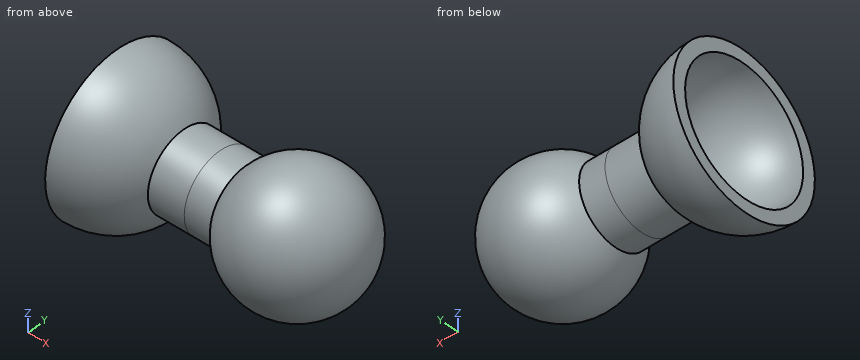
from build123d import *

# Parameters (mm, degrees)
SALIENTE_EXTRUIR2_START             = -40
CROQUIS2_R                          = 15
SALIENTE_EXTRUIR2_DEPTH             = 10
SALIENTE_EXTRUIR2_DIRECTION_2_REACH = 93.962


with BuildPart() as part:
    # Croquis1 → Revolución-Lámina1 (revolve)
    with BuildSketch(Plane(origin=(0, 0, 0), x_dir=(1, 0, 0), z_dir=(0, 1, 0))):
        with BuildLine():
            ThreePointArc((25, 0), (17.67766953, 17.67766953), (0, 25))
            Line((0, 25), (0, 30))
            ThreePointArc((0, 30), (21.213203436, 21.213203436), (30, 0))
            Line((30, 0), (25, 0))
        make_face()
    revolve(axis=Axis((0, 0, 0), (1, 0, 0)))

    # Croquis2 → Saliente-Extruir2 (add)
    with BuildSketch(Plane.ZY.offset(SALIENTE_EXTRUIR2_START)):
        Circle(CROQUIS2_R)
    extrude(amount=-SALIENTE_EXTRUIR2_DEPTH)

    # Croquis2 → Saliente-Extruir2 direction 2 (add, up to next)
    with BuildSketch(Plane.ZY.offset(SALIENTE_EXTRUIR2_START), mode=Mode.PRIVATE) as saliente_extruir2_direction_2_sk1:
        Circle(CROQUIS2_R)
    saliente_extruir2_direction_2_tool1 = extrude(saliente_extruir2_direction_2_sk1.sketch, amount=SALIENTE_EXTRUIR2_DIRECTION_2_REACH, mode=Mode.PRIVATE) - part.part
    add(saliente_extruir2_direction_2_tool1.solids().sort_by_distance((40, 0, 0))[0])

    # Croquis3 → Revolución1 (revolve)
    with BuildSketch(Plane.XY, mode=Mode.PRIVATE) as revoluci_n1_sk:
        with BuildLine():
            Line((50, 0), (50, 15))
            ThreePointArc((50, 15), (77.90569415, 23.717082451), (95, 0))
            Line((95, 0), (50, 0))
        make_face()
    revolve(revoluci_n1_sk.sketch.rotate(Axis((50, 0, 0), (1, 0, 0)), 90), axis=Axis((50, 0, 0), (1, 0, 0)))


solid = part.part
Source: CAD feature listing. Evaluate the final solid. Frame: model axes, mm. Round coordinates to 2 decimals unless told otherwise and drop trailing zeros. Loops run counter-clockwise (first coordinate to the right, second up) from the corner with the lowest first, then second, coordinate; pieces in that order, holes last. Notation, with made-up numbers: (16.5, -12.5) - (64.5, -12.5) arc R20 ccw to (64.5, -3.5) - close; hole circle Ø8 at (53.25, 13.25). An arc over 180 degrees is marked (long way). Write item = value, one per line. Start each with the question number.
(1) Section query C-C, the plane z = 20.5. Output: boundary loops of the cut face in (x, y).
(2) Section query D-D, the plane y = -17. Output: boundary loops of the cut face in (x, z), plus the area to 3 significant figures.
(3) Pin query (flat end, axial travel): pin 1 (5 mm diameter, centred on x = 28, y = 13, fed in from +Z); pin 2 (1 mm diameter, centred on y = -13.5, z = 18, fed in from -X); pin 3 (8 mm diameter, centred on x = 75, z = -12.5, fed in from -Y). Return the tip coordinate at first contact, or that it passes through.
(4) Section query A-A, the plane y = 0. Output: boundary loops of the cut face in (x, z), plus the area to 3 significant figures.
(5) Ray query, line 1 along X through (y, z) = (-17, -1); line 2 along Y through (x, z) = (8, -20.5); line 3 along X through (y, z) = (-16.5, 7.5). Return the intervals inside material, ascending. Write a range as from..to.
Conclusion:
q1.outline = (0, -21.9) arc R21.9 ccw to (0, 21.9) - (0, 14.31) arc R14.31 cw to (0, -14.31) - close; circle Ø28.62 at (70, 0)
q2.outline = (0, -24.72) arc R24.72 ccw to (0, 24.72) - (0, 18.33) arc R18.33 cw to (0, -18.33) - close; circle Ø36.66 at (70, 0)
q2.area = 1,490 mm2
q3.pin_1 = 10.71
q3.pin_2 = 9.8
q3.pin_3 = -23.14
q4.outline = (0, -30) arc R30 ccw to (25.98, -15) - (50, -15) arc R25 ccw (long way) to (50, 15) - (25.98, 15) arc R30 ccw to (0, 30) - (0, 25) arc R25 cw to (0, -25) - close
q4.area = 2,930 mm2
q5.line_1 = 18.3..24.7, 51.7..88.3
q5.line_2 = -20.39..-11.86, 11.86..20.39
q5.line_3 = 17.22..23.91, 52.78..87.22
